Can you work these out from the model? Positions are in its coordinate system, mm. Face numbers are marked on the shaded views. A direction names the side the tool comes from. Round coordinates to 2 decimals unless told otherwise and drop trailing zeros.
from build123d import *

# Parameters (mm, degrees)
F1_DEPTH = 2.2
F2_DEPTH = 3.2


with BuildPart() as f1:
    # F0 (on Top) → F1 (new body)
    with BuildSketch(Plane.XY):
        with BuildLine():
            ThreePointArc((47.0567276318, 18.8773899614), (50.5400845213, 24.8992537865), (51.75, 31.75))
            ThreePointArc((51.75, 31.75), (48.1739643306, 43.1628609764), (38.7246604334, 50.4944421586))
            add(Edge.make_bspline(
                [(38.7246604334, 50.4944421586), (38.9609346181, 49.9686786288), (41.6774554399, 43.8176291657), (44.2250191929, 36.4340414246), (46.6159564174, 23.5665925252), (47.0567276318, 18.8773899614)],
                knots=[0.630442373, 0.630442373, 0.630442373, 0.630442373, 0.6456439018, 0.8103538291, 0.929794225, 0.929794225, 0.929794225, 0.929794225], degree=3))
        make_face()
        with BuildLine():
            add(Edge.make_bspline(
                [(38.7246604334, 50.4944421586), (38.9609346181, 49.9686786288), (41.6774554399, 43.8176291657), (44.2250191929, 36.4340414246), (46.6159564174, 23.5665925252), (47.0567276318, 18.8773899614)],
                knots=[0.630442373, 0.630442373, 0.630442373, 0.630442373, 0.6456439018, 0.8103538291, 0.929794225, 0.929794225, 0.929794225, 0.929794225], degree=3))
            ThreePointArc((38.7246604334, 50.4944421586), (31.5618373499, 51.7491148508), (24.4238894806, 50.3598926557))
            add(Edge.make_bspline(
                [(15.7865923671, 19.7013645276), (16.2278990367, 23.0877163293), (18.1065072741, 32.7418176771), (22.097534659, 44.5584231861), (24.4238894806, 50.3598926557)],
                knots=[0.0983218299, 0.0983218299, 0.0983218299, 0.0983218299, 0.1865319985, 0.3205820871, 0.3205820871, 0.3205820871, 0.3205820871], degree=3))
            ThreePointArc((15.7865923672, 19.7013645276), (17.2967492534, 17.9259794974), (19.0032017299, 16.3383442206))
            add(Edge.make_bspline(
                [(19.0032017299, 16.3383442206), (20.8233538612, 19.3366897096), (25.818648602, 26.6169979909), (33.4803777859, 30.0196222141), (36.5823023021, 30.7882130146)],
                knots=[0.2222997297, 0.2222997297, 0.2222997297, 0.2222997297, 0.5388931801, 1, 1, 1, 1], degree=3))
            add(Edge.make_bspline(
                [(45.0616821781, 16.8235430329), (44.1054826127, 19.0614489649), (41.7058120017, 24.2306114406), (38.7451071997, 29.2835529549), (36.5823023021, 30.7882130146)],
                knots=[0.2242106798, 0.2242106798, 0.2242106798, 0.2242106798, 0.5365477963, 1, 1, 1, 1], degree=3))
            ThreePointArc((45.0616821781, 16.8235430329), (46.0960069989, 17.8147180442), (47.0567276318, 18.8773899614))
        make_face()
        with BuildLine():
            ThreePointArc((24.4238894806, 50.3598926557), (31.5618373499, 51.7491148508), (38.7246604334, 50.4944421586))
            add(Edge.make_bspline(
                [(24.4238894806, 50.3598926557), (25.9905275085, 54.2667784859), (28.8395118431, 60.4223481909), (32.1998298153, 63.8051247243), (36.5212033159, 55.3976328882), (38.7246604334, 50.4944421586)],
                knots=[0.3205820871, 0.3205820871, 0.3205820871, 0.3205820871, 0.4108554902, 0.4886752267, 0.630442373, 0.630442373, 0.630442373, 0.630442373], degree=3))
        make_face()
        with BuildLine():
            add(Edge.make_bspline(
                [(47.0567276318, 18.8773899614), (47.3158081923, 16.1211273275), (47.379945731, 13.6134596383), (47.1355328849, 11.710731416)],
                knots=[0.929794225, 0.929794225, 0.929794225, 0.929794225, 1, 1, 1, 1], degree=3))
            ThreePointArc((47.0567276318, 18.8773899614), (46.0960069989, 17.8147180442), (45.0616821781, 16.8235430329))
            add(Edge.make_bspline(
                [(47.1355328849, 11.710731416), (46.4293822406, 13.5298032206), (45.7480884465, 15.2170659798), (45.0616821781, 16.8235430329)],
                knots=[0, 0, 0, 0, 0.2242106798, 0.2242106798, 0.2242106798, 0.2242106798], degree=3))
        make_face()
        with BuildLine():
            add(Edge.make_bspline(
                [(15.7865923671, 19.7013645276), (16.2278990367, 23.0877163293), (18.1065072741, 32.7418176771), (22.097534659, 44.5584231861), (24.4238894806, 50.3598926557)],
                knots=[0.0983218299, 0.0983218299, 0.0983218299, 0.0983218299, 0.1865319985, 0.3205820871, 0.3205820871, 0.3205820871, 0.3205820871], degree=3))
            ThreePointArc((24.4238894806, 50.3598926557), (12.4993701223, 37.1733983178), (15.7865923672, 19.7013645276))
        make_face()
        with BuildLine():
            ThreePointArc((19.0032017299, 16.3383442206), (32.1223277175, 11.7534659986), (45.0616821781, 16.8235430329))
            add(Edge.make_bspline(
                [(45.0616821781, 16.8235430329), (44.1054826127, 19.0614489649), (41.7058120017, 24.2306114406), (38.7451071997, 29.2835529549), (36.5823023021, 30.7882130146)],
                knots=[0.2242106798, 0.2242106798, 0.2242106798, 0.2242106798, 0.5365477963, 1, 1, 1, 1], degree=3))
            add(Edge.make_bspline(
                [(19.0032017299, 16.3383442206), (20.8233538612, 19.3366897096), (25.818648602, 26.6169979909), (33.4803777859, 30.0196222141), (36.5823023021, 30.7882130146)],
                knots=[0.2222997297, 0.2222997297, 0.2222997297, 0.2222997297, 0.5388931801, 1, 1, 1, 1], degree=3))
        make_face()
        with BuildLine():
            ThreePointArc((19.0032017299, 16.3383442206), (17.2967492534, 17.9259794974), (15.7865923672, 19.7013645276))
            add(Edge.make_bspline(
                [(15.4055802766, 10.1816686965), (15.180831424, 12.7053480538), (15.2946980654, 15.9268302417), (15.7865923671, 19.7013645276)],
                knots=[0, 0, 0, 0, 0.0983218299, 0.0983218299, 0.0983218299, 0.0983218299], degree=3))
            add(Edge.make_bspline(
                [(15.4055802766, 10.1816686965), (16.5523225946, 12.1106349554), (17.7251609925, 14.2330214765), (19.0032017299, 16.3383442206)],
                knots=[0, 0, 0, 0, 0.2222997297, 0.2222997297, 0.2222997297, 0.2222997297], degree=3))
        make_face()
    extrude(amount=F1_DEPTH)

    # F0 (on Top) → F2 (join)
    with BuildSketch(Plane.XY):
        with BuildLine():
            add(Edge.make_bspline(
                [(38.7246604334, 50.4944421586), (38.9609346181, 49.9686786288), (41.6774554399, 43.8176291657), (44.2250191929, 36.4340414246), (46.6159564174, 23.5665925252), (47.0567276318, 18.8773899614)],
                knots=[0.630442373, 0.630442373, 0.630442373, 0.630442373, 0.6456439018, 0.8103538291, 0.929794225, 0.929794225, 0.929794225, 0.929794225], degree=3))
            ThreePointArc((38.7246604334, 50.4944421586), (31.5618373499, 51.7491148508), (24.4238894806, 50.3598926557))
            add(Edge.make_bspline(
                [(15.7865923671, 19.7013645276), (16.2278990367, 23.0877163293), (18.1065072741, 32.7418176771), (22.097534659, 44.5584231861), (24.4238894806, 50.3598926557)],
                knots=[0.0983218299, 0.0983218299, 0.0983218299, 0.0983218299, 0.1865319985, 0.3205820871, 0.3205820871, 0.3205820871, 0.3205820871], degree=3))
            ThreePointArc((15.7865923672, 19.7013645276), (17.2967492534, 17.9259794974), (19.0032017299, 16.3383442206))
            add(Edge.make_bspline(
                [(19.0032017299, 16.3383442206), (20.8233538612, 19.3366897096), (25.818648602, 26.6169979909), (33.4803777859, 30.0196222141), (36.5823023021, 30.7882130146)],
                knots=[0.2222997297, 0.2222997297, 0.2222997297, 0.2222997297, 0.5388931801, 1, 1, 1, 1], degree=3))
            add(Edge.make_bspline(
                [(45.0616821781, 16.8235430329), (44.1054826127, 19.0614489649), (41.7058120017, 24.2306114406), (38.7451071997, 29.2835529549), (36.5823023021, 30.7882130146)],
                knots=[0.2242106798, 0.2242106798, 0.2242106798, 0.2242106798, 0.5365477963, 1, 1, 1, 1], degree=3))
            ThreePointArc((45.0616821781, 16.8235430329), (46.0960069989, 17.8147180442), (47.0567276318, 18.8773899614))
        make_face()
        with BuildLine():
            ThreePointArc((24.4238894806, 50.3598926557), (31.5618373499, 51.7491148508), (38.7246604334, 50.4944421586))
            add(Edge.make_bspline(
                [(24.4238894806, 50.3598926557), (25.9905275085, 54.2667784859), (28.8395118431, 60.4223481909), (32.1998298153, 63.8051247243), (36.5212033159, 55.3976328882), (38.7246604334, 50.4944421586)],
                knots=[0.3205820871, 0.3205820871, 0.3205820871, 0.3205820871, 0.4108554902, 0.4886752267, 0.630442373, 0.630442373, 0.630442373, 0.630442373], degree=3))
        make_face()
        with BuildLine():
            add(Edge.make_bspline(
                [(47.0567276318, 18.8773899614), (47.3158081923, 16.1211273275), (47.379945731, 13.6134596383), (47.1355328849, 11.710731416)],
                knots=[0.929794225, 0.929794225, 0.929794225, 0.929794225, 1, 1, 1, 1], degree=3))
            ThreePointArc((47.0567276318, 18.8773899614), (46.0960069989, 17.8147180442), (45.0616821781, 16.8235430329))
            add(Edge.make_bspline(
                [(47.1355328849, 11.710731416), (46.4293822406, 13.5298032206), (45.7480884465, 15.2170659798), (45.0616821781, 16.8235430329)],
                knots=[0, 0, 0, 0, 0.2242106798, 0.2242106798, 0.2242106798, 0.2242106798], degree=3))
        make_face()
        with BuildLine():
            ThreePointArc((19.0032017299, 16.3383442206), (17.2967492534, 17.9259794974), (15.7865923672, 19.7013645276))
            add(Edge.make_bspline(
                [(15.4055802766, 10.1816686965), (15.180831424, 12.7053480538), (15.2946980654, 15.9268302417), (15.7865923671, 19.7013645276)],
                knots=[0, 0, 0, 0, 0.0983218299, 0.0983218299, 0.0983218299, 0.0983218299], degree=3))
            add(Edge.make_bspline(
                [(15.4055802766, 10.1816686965), (16.5523225946, 12.1106349554), (17.7251609925, 14.2330214765), (19.0032017299, 16.3383442206)],
                knots=[0, 0, 0, 0, 0.2222997297, 0.2222997297, 0.2222997297, 0.2222997297], degree=3))
        make_face()
    extrude(amount=F2_DEPTH)


solid = f1.part
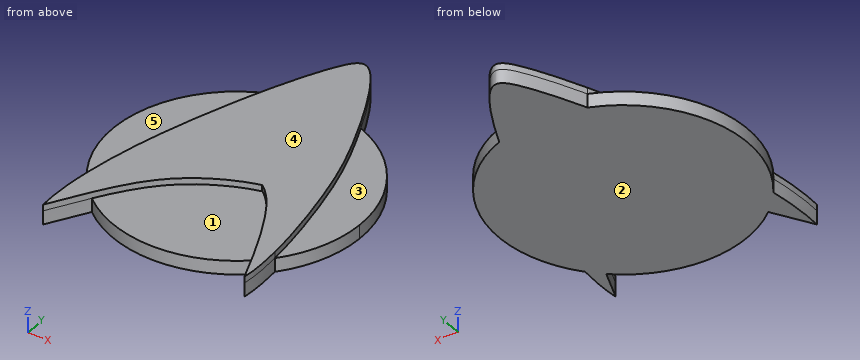
(1) For the marked faces 3, 4 and 5, which set-ups out of +Z, -Z, +X, -X, +Y, -Y let a thin tool reach every point of the face, with its end or its side?
Worked answers:
face 3: +Z, +X, +Y
face 4: +Z, +X, -X, +Y, -Y
face 5: +Z, -X, +Y
(2) If I drill on line 1 (Z direction, x = 13, y = 34); line 2 (X direction, y = 15.5, z = 2.9); line 3 (X direction, y = 53, z = 2.7), over which ranges is the centre line in solid material (lowest first)?
Worked answers:
line 1: z = 0 to 2.2
line 2: x = 15.38 to 18.5, 45.62 to 47.27
line 3: x = 25.52 to 37.56
(3) Will this pin go through, and if not, where does the flat tip stop? P1, Ø1.5, axis at y = 15.5, z = 3, coming from the -X side.
Worked answers:
P1: stops at x = 15.34
(4) If we section it at A-A, the plane y = 14.5: State how many separate pieces and enclosed holes the cut face has, then the cut area to 3 significant figures.
Worked answers:
separate pieces: 3
enclosed holes: 0
area: 56.8 mm2
(5) If we mould it in two halves opening along X, with no side actions, what happens to the marked faces 1 and 2? For each: released by +X, released by -X, zero draft, split by the parting line, or undercut.
Worked answers:
face 1: undercut
face 2: zero draft
